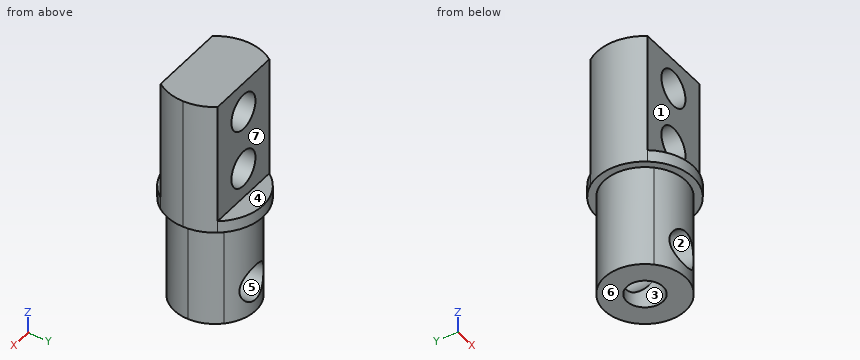
```python
from build123d import *

# Parameters (mm, degrees)
SKETCH1_R               = 2.3876
EXTRUDE1_DEPTH          = 17.47
EXTRUDE2_DEPTH          = 1.5875
SKETCH1_4_R             = 2.3876
EXTRUDE3_DEPTH          = 13.487
CUT_EXTRUDE1_START      = -3.9624
SKETCH1_5_R             = 2.3876
CUT_EXTRUDE1_DEPTH      = 13.487
SKETCH2_R               = 2.3813
CUT_EXTRUDE2_DEPTH      = 13.487
CUT_EXTRUDE2_DEPTH_BACK = 13.487


with BuildPart() as part:
    # Sketch1 → Extrude1 (new body)
    with BuildSketch(Plane.XY):
        with BuildLine():
            Line((3.829692416, 3.7465), (-3.829692416, 3.7465))
            ThreePointArc((-3.829692416, 3.7465), (-5.3575, 0), (-3.829692416, -3.7465))
            Line((-3.829692416, -3.7465), (3.829692416, -3.7465))
            ThreePointArc((3.829692416, -3.7465), (4.960866022, -2.023021148), (5.3575, 0))
            ThreePointArc((5.3575, 0), (4.960866022, 2.023021148), (3.829692416, 3.7465))
        make_face()
        Circle(SKETCH1_R, mode=Mode.SUBTRACT)
        with BuildLine():
            Line((-3.829692416, 3.7465), (-5.127010606, 3.7465))
            ThreePointArc((-5.127010606, 3.7465), (-6.35, 0), (-5.127010606, -3.7465))
            Line((-5.127010606, -3.7465), (-3.829692416, -3.7465))
            ThreePointArc((-3.829692416, -3.7465), (-5.3575, 0), (-3.829692416, 3.7465))
        make_face()
        with BuildLine():
            ThreePointArc((6.35, 0), (6.036514613, 1.970530722), (5.127010606, 3.7465))
            Line((5.127010606, 3.7465), (3.829692416, 3.7465))
            ThreePointArc((3.829692416, 3.7465), (4.960866022, 2.023021148), (5.3575, 0))
            ThreePointArc((5.3575, 0), (4.960866022, -2.023021148), (3.829692416, -3.7465))
            Line((3.829692416, -3.7465), (5.127010606, -3.7465))
            ThreePointArc((5.127010606, -3.7465), (6.036514613, -1.970530722), (6.35, 0))
        make_face()
        with BuildLine():
            Line((-3.829692416, 3.7465), (-5.127010606, 3.7465))
            ThreePointArc((-5.127010606, 3.7465), (-6.35, 0), (-5.127010606, -3.7465))
            Line((-5.127010606, -3.7465), (-3.829692416, -3.7465))
            ThreePointArc((-3.829692416, -3.7465), (-5.3575, 0), (-3.829692416, 3.7465))
        make_face()
        with BuildLine():
            ThreePointArc((6.35, 0), (6.036514613, 1.970530722), (5.127010606, 3.7465))
            Line((5.127010606, 3.7465), (3.829692416, 3.7465))
            ThreePointArc((3.829692416, 3.7465), (4.960866022, 2.023021148), (5.3575, 0))
            ThreePointArc((5.3575, 0), (4.960866022, -2.023021148), (3.829692416, -3.7465))
            Line((3.829692416, -3.7465), (5.127010606, -3.7465))
            ThreePointArc((5.127010606, -3.7465), (6.036514613, -1.970530722), (6.35, 0))
        make_face()
        Circle(SKETCH1_R)
    extrude(amount=EXTRUDE1_DEPTH)

    # Sketch1_3 → Extrude2 (add)
    with BuildSketch(Plane.XY):
        with BuildLine():
            ThreePointArc((5.127010606, 3.7465), (0, 6.35), (-5.127010606, 3.7465))
            Line((-5.127010606, 3.7465), (-3.829692416, 3.7465))
            ThreePointArc((-3.829692416, 3.7465), (0, 5.3575), (3.829692416, 3.7465))
            Line((3.829692416, 3.7465), (5.127010606, 3.7465))
        make_face()
        with BuildLine():
            ThreePointArc((3.829692416, 3.7465), (0, 5.3575), (-3.829692416, 3.7465))
            Line((-3.829692416, 3.7465), (3.829692416, 3.7465))
        make_face()
        with BuildLine():
            Line((-3.829692416, -3.7465), (-5.127010606, -3.7465))
            ThreePointArc((-5.127010606, -3.7465), (0, -6.35), (5.127010606, -3.7465))
            Line((5.127010606, -3.7465), (3.829692416, -3.7465))
            ThreePointArc((3.829692416, -3.7465), (0, -5.3575), (-3.829692416, -3.7465))
        make_face()
        with BuildLine():
            Line((3.829692416, -3.7465), (-3.829692416, -3.7465))
            ThreePointArc((-3.829692416, -3.7465), (0, -5.3575), (3.829692416, -3.7465))
        make_face()
    extrude(amount=EXTRUDE2_DEPTH)

    # Sketch1_4 → Extrude3 (add)
    with BuildSketch(Plane.XY):
        with BuildLine():
            Line((3.829692416, 3.7465), (-3.829692416, 3.7465))
            ThreePointArc((-3.829692416, 3.7465), (-5.3575, 0), (-3.829692416, -3.7465))
            Line((-3.829692416, -3.7465), (3.829692416, -3.7465))
            ThreePointArc((3.829692416, -3.7465), (4.960866022, -2.023021148), (5.3575, 0))
            ThreePointArc((5.3575, 0), (4.960866022, 2.023021148), (3.829692416, 3.7465))
        make_face()
        Circle(SKETCH1_4_R, mode=Mode.SUBTRACT)
        Circle(SKETCH1_4_R)
        with BuildLine():
            Line((3.829692416, -3.7465), (-3.829692416, -3.7465))
            ThreePointArc((-3.829692416, -3.7465), (0, -5.3575), (3.829692416, -3.7465))
        make_face()
        with BuildLine():
            ThreePointArc((3.829692416, 3.7465), (0, 5.3575), (-3.829692416, 3.7465))
            Line((-3.829692416, 3.7465), (3.829692416, 3.7465))
        make_face()
    extrude(amount=-EXTRUDE3_DEPTH)

    # Sketch1_5 → Cut-Extrude1 (cut)
    with BuildSketch(Plane.XY.offset(CUT_EXTRUDE1_START)):
        Circle(SKETCH1_5_R)
    extrude(amount=-CUT_EXTRUDE1_DEPTH, mode=Mode.SUBTRACT)

    # Sketch2 → Cut-Extrude2 (cut, two sides)
    with BuildSketch(Plane(origin=(0, 0, 0), x_dir=(1, 0, 0), z_dir=(0, 1, 0))) as cut_extrude2_sk:
        with Locations(Location((0, -5.5828, 0), (0, 0, 270))):  # turned: the seam where the file's is
            Circle(SKETCH2_R)
        with Locations(Location((0, -13.4822, 0), (0, 0, 270))):  # turned: the seam where the file's is
            Circle(SKETCH2_R)
        with Locations(Location((0, 9.5175, 0), (0, 0, 270))):  # turned: the seam where the file's is
            Circle(SKETCH2_R)
    extrude(amount=CUT_EXTRUDE2_DEPTH, mode=Mode.SUBTRACT)
    extrude(cut_extrude2_sk.sketch, amount=-CUT_EXTRUDE2_DEPTH_BACK, mode=Mode.SUBTRACT)


solid = part.part
```
Geometry check sheet. Reference: the model listing, model coordinates, mm. Face numbers are marked on the shaded views. A direction names the side the tool comes from. Give positions to 0.01 mm unless a question says otherwise; leave off trailing zeros. Loops run counter-clockwise (first coordinate to the right, second up) from the corner with the lowest first, then second, coordinate; pieces in that order, holes last. Notation, with made-up numbers: M 11.5,-25 L 44.5,-25 A22 ccw 44.5,0 Z; hole C 27.25,58.25 d9. An arc over 180 degrees is marked long. Write item = value, one per line. Start each with the question number.
1. Draft check along Z on the marked faces 4, 5, 6 and 7. Enter one of: +Z half, -Z half, draft (parallel to the pull), parting line (faces both ways), or undercut.
2. Section check C-C, the plane z = -2.5. Enter the section's corners in (x, y) (1 decimal), plus the area to 3 significant figures.
3. Section check B-B, the plane z = 6. Enter the section's corners in (x, y), plus the area to 3 significant figures.
4. Section check D-D, the plane y = -0.75. Enter the section's corners in (x, z).
5. Go/stop test with flat-tipped pins: P1, Ø5.5, axis at x = 0, z = 13.48, coming from the -Y side; P2, Ø6, axis at x = 0, z = 5.58, coming from the +Y side; P3, Ø1, axis at x = -3, z = -6, coming from the -Y side. Record where each tip stops, or that it passes through.
6. Tool access check on the marked faces 1, 2 and 3. Record the directions out of +Z, -Z, +X, -X, +Y, -Y that give a thin tool (end or side, any length) a straight path to the whole face; none if there is none.
7. Section check A-A, the plane x = 0. Give the number of separate pieces and of enclosed holes in the cut face, plus the area to 3 significant figures.
8. Thickness scan on probe 1 along Z at (x, y) = (0, 2.65); probe 2 along Z at (x, y) = (0, 2.3); probe 3 along Z at (x, y) = (1, 1). Record the ranges inside material, lowest first.
Values follow:
q1.face_4 = +Z half
q1.face_5 = undercut
q1.face_6 = -Z half
q1.face_7 = draft
q2.outline = C 0,0 d10.7
q2.area = 90.2 mm^2
q3.outline = M -5.13,-3.75 L -2.34,-3.75 L -2.34,3.75 L -5.13,3.75 A6.35 ccw Z; M 2.34,-3.75 L 5.13,-3.75 A6.35 ccw 5.13,3.75 L 2.34,3.75 Z
q3.area = 54.2 mm^2
q4.outline = M -6.31,0 L -5.3,0 L -5.3,-13.49 L -2.27,-13.49 L -2.27,-10.25 A2.38 cw -2.27,-8.79 L -2.27,-3.96 L 2.27,-3.96 L 2.27,-8.79 A2.38 cw 2.27,-10.25 L 2.27,-13.49 L 5.3,-13.49 L 5.3,0 L 6.31,0 L 6.31,17.47 L -6.31,17.47 Z; hole C 0,5.58 d4.76; hole C 0,13.48 d4.76
q5.P1 = -3.75
q5.P2 = 3.75
q5.P3 = -4.74
q6.face_1 = +Z, +X, -X, -Y
q6.face_2 = +Y, -Y
q6.face_3 = -Z
q7.separate_pieces = 5
q7.enclosed_holes = 0
q7.area = 139 mm^2
q8.probe_1 = -13.49 to -11.9, -7.14 to 3.2, 7.96 to 11.1, 15.86 to 17.47
q8.probe_2 = -3.96 to 3.2, 7.96 to 11.1, 15.86 to 17.47
q8.probe_3 = -3.96 to 3.42, 7.74 to 11.32, 15.64 to 17.47
